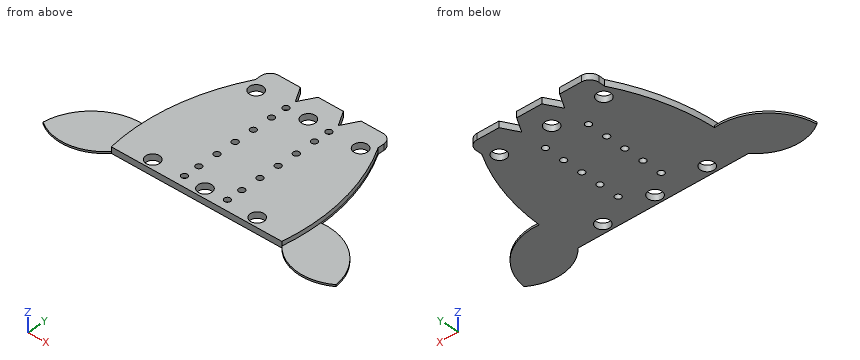
Autodesk Inventor part; units mm, degrees
ref_plane "YZ Plane" through (0, 0, 0) normal (1, 0, 0) x (0, 1, 0)
ref_plane "XZ Plane" through (0, 0, 0) normal (0, 1, 0) x (-1, 0, 0)
ref_plane "XY Plane" through (0, 0, 0) normal (0, 0, 1) x (1, 0, 0)
sketch "Block1" plane through (0, 0, 0) normal (0, 0, 1) x (1, 0, 0)
  line L0 (22.5674, 54.9733) -> (22.5674, 26.9733) construction
  line L1 (62.5674, 54.9733) -> (62.5674, 26.9733) construction
  line L2 (42.5674, 54.9733) -> (42.5674, 26.9733) construction
  arc A0 (22.5674, 54.9733) -> (16.0189, 31.9733) centre (39.6923, 37.6653) ccw
  arc A1 (69.116, 31.9733) -> (62.5674, 54.9733) centre (45.4425, 37.6653) ccw
  line L3 (67.5674, 31.9733) -> (69.116, 31.9733)
  line L4 (22.5674, 54.9733) -> (62.5674, 54.9733)
  arc A2 (3.175, 28.049) -> (16.0189, 31.9733) centre (7.7246, 36.1392) ccw
  arc A3 (15.3685, 38.7512) -> (3.175, 28.049) centre (13.5542, 28.5209) ccw
  arc A4 (69.116, 31.9733) -> (81.9598, 28.049) centre (77.4102, 36.1392) ccw
  arc A5 (81.9598, 28.049) -> (69.7664, 38.7512) centre (71.5807, 28.5209) ccw
  line L5 (17.5674, 54.9733) -> (67.5674, 54.9733) construction
  line L6 (67.5674, 54.9733) -> (67.5674, 31.9733) construction
  line L7 (67.5674, 31.9733) -> (16.0189, 31.9733)
  line L8 (17.5674, 31.9733) -> (17.5674, 54.9733) construction
  line L9 (22.5674, 31.9733) -> (62.5674, 31.9733)
  line L10 (62.5674, 31.9733) -> (62.5674, 26.9733)
  line L11 (62.5674, 26.9733) -> (22.5674, 26.9733)
  line L12 (22.5674, 26.9733) -> (22.5674, 31.9733)
  circle A6 centre (35.5674, 51.6287) radius 1
  circle A7 centre (49.5674, 51.6287) radius 1
  line L13 (22.5674, 29.4733) -> (62.5674, 29.4733) construction
  circle A8 centre (35.5674, 29.4733) radius 1
  circle A9 centre (49.5674, 29.4733) radius 1
  point P0 (42.5377, 37.3132)
  point P1 (42.5674, 31.9733)
  point P2 (42.5674, 31.9733)
  point P3 (17.5674, 26.9733)
  point P4 (67.5674, 26.9733)
  dimension "d0" = 23
  dimension "d1" = 5
  dimension "d2" = 40
  dimension "d3" = 2
  dimension "d4" = 2
  dimension "d5" = 7
  dimension "d6" = 7
  dimension "d7" = 2
  dimension "d8" = 2
  dimension "d9" = 7
  dimension "d10" = 7
sketch "Sketch1" plane through (0, 0, 0) normal (0, 0, 1) x (1, 0, 0)
  line L0 (-20, 21.5) -> (-20, -26.5) construction
  line L1 (20, 21.5) -> (20, -26.5) construction
  line L2 (0, 21.5) -> (0, -26.5) construction
  arc A0 (-20, 21.5) -> (-27.7782, -21.5) centre (37.6183, -11.126) ccw
  arc A1 (27.7782, -21.5) -> (20, 21.5) centre (-37.6183, -11.126) ccw
  line L3 (25, -21.5) -> (27.7782, -21.5)
  line L4 (-20, 21.5) -> (20, 21.5)
  line L5 (-25, 21.5) -> (25, 21.5) construction
  line L6 (25, 21.5) -> (25, -21.5) construction
  line L7 (25, -21.5) -> (-27.7782, -21.5)
  line L8 (-25, -21.5) -> (-25, 21.5) construction
  line L9 (-20, -21.5) -> (20, -21.5)
  line L10 (20, -21.5) -> (20, -26.5)
  line L11 (20, -26.5) -> (-20, -26.5)
  line L12 (-20, -26.5) -> (-20, -21.5)
  circle A2 centre (-7, 18.1554) radius 1
  circle A3 centre (7, 18.1554) radius 1
  line L13 (-20, -24) -> (20, -24) construction
  circle A4 centre (-7, -24) radius 1
  circle A5 centre (7, -24) radius 1
  circle A6 centre (-17, -18.5) radius 2.25
  circle A7 centre (17, -18.5) radius 2.25
  circle A8 centre (0, -18.5) radius 2.25
  line L14 (-25, 0) -> (25, 0) construction
  line L15 (-20, 21.5) -> (20, 21.5)
  line L16 (20, 21.5) -> (20, 26.5)
  line L17 (20, 26.5) -> (-20, 26.5)
  line L18 (-20, 26.5) -> (-20, 21.5)
  line L19 (-7, 18.1554) -> (-7, 26.5) construction
  line L20 (-7, 21.5) -> (-9.8868, 26.5)
  line L21 (-9.8868, 26.5) -> (-4.1132, 26.5)
  line L22 (-4.1132, 26.5) -> (-7, 21.5)
  circle A9 centre (-7, 0) radius 1
  circle A10 centre (7, 0) radius 1
  circle A11 centre (-7, -18.1554) radius 1
  circle A12 centre (7, -18.1554) radius 1
  arc A13 (-47.7296, -24) -> (-27.7782, -21.5) centre (-39.1631, -11.5041) ccw
  arc A14 (-28.5398, -8.4011) -> (-47.7296, -24) centre (-30.1563, -26.0155) ccw
  arc A15 (27.7782, -21.5) -> (47.7296, -24) centre (39.1631, -11.5041) ccw
  arc A16 (47.7296, -24) -> (28.5398, -8.4011) centre (30.1563, -26.0155) ccw
  point P0 (0, 0)
  point P1 (0, -21.5)
  point P2 (0, -21.5)
  point P3 (-27.9814, 24.963)
  point P4 (27.9814, 24.963)
  point P5 (0, -2.5)
  point P6 (0, 0)
  dimension "d12" = 43
  dimension "d13" = 5
  dimension "d14" = 40
  dimension "d15" = 2
  dimension "d16" = 2
  dimension "d17" = 7
  dimension "d18" = 7
  dimension "d19" = 2
  dimension "d20" = 2
  dimension "d21" = 7
  dimension "d22" = 7
  dimension "d24" = 4.5
  dimension "d25" = 4.5
  dimension "d26" = 3
  dimension "d27" = 3
  dimension "d28" = 3
  dimension "d29" = 3
  dimension "d34" = 4.5
  dimension "d35" = 3
  dimension "d38" = 5
  dimension "d39" = 30
  dimension "d40" = 30
  dimension "d45" = 3.3446
  dimension "d46" = 3.3446
  dimension "d47" = 2
  dimension "d48" = 2
  dimension "d49" = 7
  dimension "d50" = 7
extrude "Extrusion1" add sketch "Sketch1" along normal blind 2 contours L4 A1 L3 L7 A0 | A6 | A7 | A8 | A9 | A10
extrude "Extrusion2" add sketch "Sketch1" along normal blind 0.6 contours L4 A1 L3 L7 A0 | A2 | A3 | A6 | A7 | A8 | A9 | A10 | A11 | A12
mirror "Mirror1" about plane through (0, 0, 0) normal (1, 0, 0) of "Extrusion2"
extrude "Extrusion3" cut sketch "Sketch1" along normal blind 5 contours A6 | A7 | A8
mirror "Mirror2" about plane through (0, 0, 0) normal (0, 1, 0) of "Extrusion3"
extrude "Extrusion4" add sketch "Sketch1" along normal blind 2 contours L18 L17 L20 L4 | L22 L17 L16 L4 | L20 L17 L22
extrude "Extrusion5" cut sketch "Sketch1" along normal blind 5 contours L20 L17 L22
extrude "Extrusion7" add sketch "Sketch1" along normal blind 0.6 contours A0 A13 A14
mirror "Mirror3" about plane through (0, 0, 0) normal (1, 0, 0) of "Extrusion5", "Extrusion7"
fillet "Fillet1" radius 3 2 edges at (-20, 26.5, 1) (20, 26.5, 1)
extrude "Extrusion8" cut sketch "Sketch1" along normal blind 10 contours A9 | A10
pattern_linear "Rectangular Pattern1" count 3 spacing 6.5 along (0, 1, 0) count 3 spacing 6.5 along (0, -1, 0) of "Extrusion8"
equation "\"d3\" = d11"
equation "\"d4\" = d11"
equation "\"d7\" = d11"
equation "\"d8\" = d11"
equation "\"d15\" = fishing"
equation "\"d16\" = fishing"
equation "\"d19\" = fishing"
equation "\"d20\" = fishing"
equation "\"d47\" = fishing"
equation "\"d48\" = fishing"
equation "\"d56\" = 2 * layer"
equation "\"d11\" = 2"
equation "\"d23\" = 2"
properties part number "Piece"
Model file for the job. Use its own axes, mm. Give positions to 0.01 mm unless a question says otherwise; leave off trailing zeros. Order: outer loops, then holes, each group sorted by start corner. A loop starts at its lowest first (then second) coordinate and runs counter-clockwise, first axis right, second up. Notation, with made-up numbers: (-7.75, -0.5) - (38.25, -0.5) arc R14 ccw to (38.25, 10.5) - close; hole circle Ø5 at (75, -28.75). An arc over 180 degrees is marked (long way). One line per item, written item: value.
Item 1: Slice it at C-C (x = 1). List the corners of the cut face in (y, z).
Response values:
outline: (-21.5, 0) - (-20.52, 0) - (-20.52, 2) - (-21.5, 2) - close; (-16.48, 0) - (16.48, 0) - (16.48, 2) - (-16.48, 2) - close; (20.52, 0) - (26.5, 0) - (26.5, 2) - (20.52, 2) - close
Item 2: Slice it at A-A (z = 1.1). Give the number of separate pieces and of enclosed holes in the cut face, then the cut area to 3 significant figures.
Response values:
separate pieces: 1
enclosed holes: 20
area: 2,300 mm2
Item 3: Pin check, flat tips, straight feed: pin 1 Ø1.2 at (x, y) = (7, 6.5) entering from +Z; pin 2 Ø1 at (x, z) = (1.5, 1) entering from -Y; pin 3 Ø1.6 at (x, y) = (7, 18.16) entering from +Z. Stop position of each tip, or through.
Response values:
pin 1: through
pin 2: y = -21.5
pin 3: z = 0.6
Item 4: Wall check: line 1 (Y direction, x = -17, z = 0.95); line 2 (X direction, y = 24, z = 1.3); line 3 (X direction, y = 16.5, z = 1.2). Give the ranges that are in metal, low to high.
Response values:
line 1: -21.5 to -20.75, -16.25 to 16.25, 20.75 to 26.5
line 2: -19.96 to -8.44, -5.56 to 5.56, 8.44 to 19.96
line 3: -22.56 to -18.03, -15.97 to -1.03, 1.03 to 15.97, 18.03 to 22.56
Item 5: Slice it at B-B (y = 0). List the corners of the cut face in (x, z), then the cut area to 3 significant figures.
Response values:
outline: (-27.65, 0) - (-8, 0) - (-8, 2) - (-27.65, 2) - close; (-6, 0) - (6, 0) - (6, 2) - (-6, 2) - close; (8, 0) - (27.65, 0) - (27.65, 2) - (8, 2) - close
area: 103 mm2
Item 6: Slice it at D-D (x = 12). List the corners of the cut face in (y, z), then the cut area to 3 significant figures.
Response values:
outline: (-21.5, 0) - (26.5, 0) - (26.5, 2) - (-21.5, 2) - close
area: 96.0 mm2
